The figure shows three views and two pictorial views of one solid part (mm, origin at its lowest corner). Answer the questions. A direction names the side the tool comes from. Give positions to 0.01 mm unless a question says otherwise; leave off trailing zeros. Order: outer loops, then holes, each group sorted by start corner. A loop starts at its lowest first (then second) coordinate and runs counter-clockwise, first axis right, second up. Notation, with made-up numbers: (43, 3) - (61, 3) arc R7 cw to (61, 13) - close; hole circle Ø1 at (54.5, -12.75). An arc over 180 degrees is marked (long way). Answer as a JSON object with one key per item and string values. Group by question number.
Q1. Consider line 1 (Y direction, x = 25, z = 2.25); line 2 (Z direction, x = 29.5, y = 8.5); line 3 (Y direction, x = 25, z = 47). Determine where each line is inside the solid, lowest interval first.
Q2. A cutting plane is placed at C-C, the plane x = 4. Give the vertices of the cut face in (y, z) (1 decimal).
Q3. Given pin 1 (3 mm diameter, centred on x = 23.5, z = 34.5, fed in from +Y); pin 2 (1 mm diameter, centred on y = 24, z = 22, fed in from +X); pin 3 (5 mm diameter, centred on y = 13.5, z = 51, fed in from +X); pin 4 (7 mm diameter, centred on x = 25, y = 25, fed in from +Z), each flat-ended and moving along its own axis, determine where each tip first touches the part or whether it passes through.
Q4. A cutting plane is placed at D-D, the plane z = 39. Give the vertices of the cut face in (x, y).
Q5. A cutting plane is placed at A-A, the plane x = 25. Give the vertices of the cut face in (y, z).
Q6. A cutting plane is placed at B-B, the plane y = 25. Give the vertices of the cut face in (x, z), and give its area (3 significant figures).
Q7. For the marked faces 1 and 2, determine the directions among +Z, -Z, +X, -X, +Y, -Y from which every point of the face is accessible in a straight line to the end or side of a thin tool.
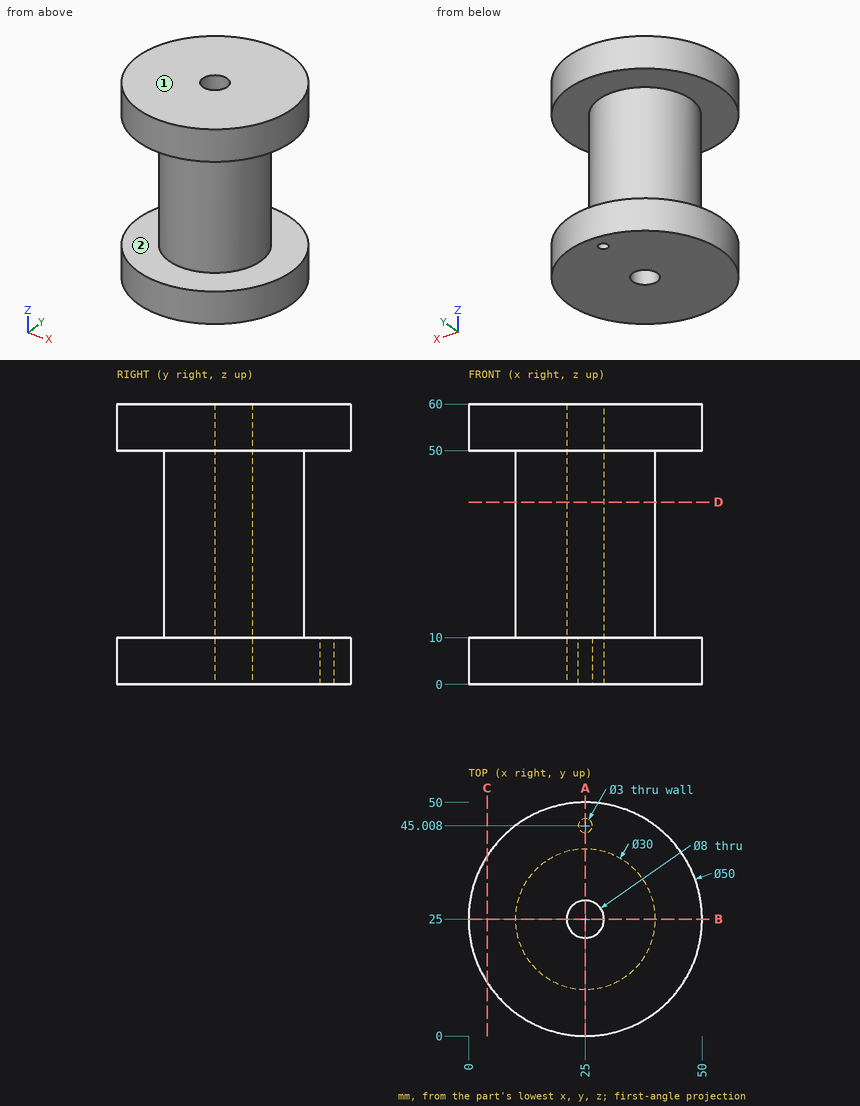
Reply:
{
 "1": {"line 1": "y = 0 to 21, 29 to 43.51, 46.51 to 50", "line 2": "z = 0 to 10, 50 to 60", "line 3": "y = 10 to 21, 29 to 40"},
 "2": {"outline": "(11.4, 0) - (38.6, 0) - (38.6, 10) - (11.4, 10) - close; (11.4, 50) - (38.6, 50) - (38.6, 60) - (11.4, 60) - close"},
 "3": {"pin 1": "stops at y = 40", "pin 2": "stops at x = 39.99", "pin 3": "stops at x = 48.32", "pin 4": "passes through"},
 "4": {"outline": "circle Ø30 at (25, 25); hole circle Ø8 at (25, 25)"},
 "5": {"outline": "(0, 0) - (21, 0) - (21, 60) - (0, 60) - (0, 50) - (10, 50) - (10, 10) - (0, 10) - close; (29, 0) - (43.51, 0) - (43.51, 10) - (40, 10) - (40, 50) - (50, 50) - (50, 60) - (29, 60) - close; (46.51, 0) - (50, 0) - (50, 10) - (46.51, 10) - close"},
 "6": {"outline": "(0, 0) - (21, 0) - (21, 60) - (0, 60) - (0, 50) - (10, 50) - (10, 10) - (0, 10) - close; (29, 0) - (50, 0) - (50, 10) - (40, 10) - (40, 50) - (50, 50) - (50, 60) - (29, 60) - close", "area": "1,720 mm^2"},
 "7": {"face 1": "+Z, +X, -X, +Y, -Y", "face 2": "none"}
}
